The model under review builds one solid part; all positions refer to its coordinate system, in mm. Face numbers are marked on the shaded views. A direction names the side the tool comes from. Round coordinates to 2 decimals unless told otherwise and drop trailing zeros. Write each loop counter-clockwise with the first axis right and the second up, starting at its lowest first coordinate (ties: lowest second). Pieces come first, ordered by that corner, then holes. Notation, with made-up numbers: (46.25, -16) - (91.25, -16) arc R19 ccw to (91.25, 8) - close; hole circle Ø8 at (6, -24.75). An arc over 180 degrees is marked (long way). Return JSON: item names as keys, results as strings.
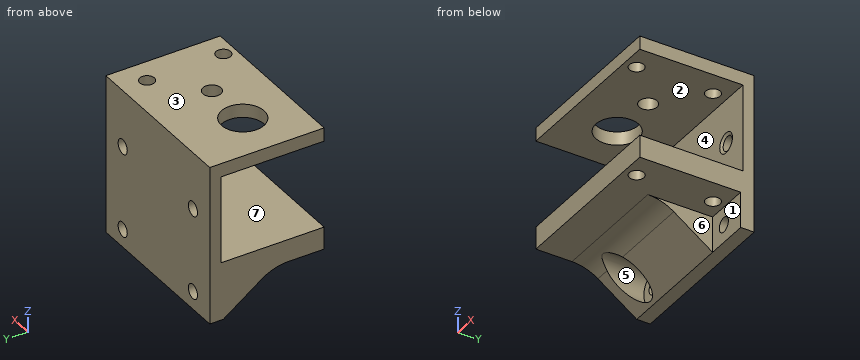
from build123d import *

# Parameters (mm, degrees)
BOSS_EXTRUDE1_OUTLINE_W   = 37
BOSS_EXTRUDE1_OUTLINE_H   = 22.5
BOSS_EXTRUDE1_OUTLINE_R   = 1.625
BOSS_EXTRUDE1_OUTLINE_R_2 = 4.75
BOSS_EXTRUDE1_OUTLINE_R_3 = 2
BOSS_EXTRUDE1_DEPTH       = 3
SKETCH2_W                 = 37
SKETCH2_H                 = 22.5
SKETCH2_R                 = 1.625
BOSS_EXTRUDE2_DEPTH       = 5
SKETCH3_W                 = 37
SKETCH3_H                 = 35.5
BOSS_EXTRUDE3_DEPTH       = 3
BOSS_EXTRUDE4_DEPTH       = 37
CUT_EXTRUDE1_DEPTH        = 10
CUT_EXTRUDE2_REACH        = 57.457
SKETCH7_R                 = 1.625
CHAMFER1_SIZE             = 1.5
CHAMFER1_SIZE2            = 0.866025404
FILLET1_R                 = 10
SKETCH8_R                 = 3.5
CUT_EXTRUDE3_DEPTH        = 22.5
SKETCH9_W                 = 37
SKETCH9_H                 = 19.5
CUT_EXTRUDE4_DEPTH        = 0.5


# Read off the part's stored shape, not the designer's step: Boss-Extrude1
with BuildPart() as part:
    # Boss-Extrude1 outline → Boss-Extrude1 (new body)
    with BuildSketch(Plane.XY):
        with Locations((18.5, 11.25)):
            Rectangle(BOSS_EXTRUDE1_OUTLINE_W, BOSS_EXTRUDE1_OUTLINE_H)
        with Locations((31.5, 2.75)):
            Circle(BOSS_EXTRUDE1_OUTLINE_R, mode=Mode.SUBTRACT)
        with Locations((11, 11.25)):
            Circle(BOSS_EXTRUDE1_OUTLINE_R_2, mode=Mode.SUBTRACT)
        with Locations((22, 11.25)):
            Circle(BOSS_EXTRUDE1_OUTLINE_R_3, mode=Mode.SUBTRACT)
        with Locations((31.5, 19.75)):
            Circle(BOSS_EXTRUDE1_OUTLINE_R, mode=Mode.SUBTRACT)
    extrude(amount=BOSS_EXTRUDE1_DEPTH)



with BuildPart() as body_2:
    # Sketch2 → Boss-Extrude2 (new body)
    with BuildSketch(Plane(origin=(0, 0, -19.5), x_dir=(-1, 0, 0), z_dir=(0, 0, -1))):
        with Locations((-18.5, 11.25)):
            Rectangle(SKETCH2_W, SKETCH2_H)
        with Locations((-31.5, 2.75)):
            Circle(SKETCH2_R, mode=Mode.SUBTRACT)
        with Locations(Location((-31.5, 19.75, 0), (0, 0, 180))):
            Circle(SKETCH2_R, mode=Mode.SUBTRACT)
    extrude(amount=BOSS_EXTRUDE2_DEPTH)


with BuildPart() as part_1:
    add(part.part)

    add(body_2.part)  # Boss-Extrude3 merges body 2
    # Sketch3 → Boss-Extrude3 (add)
    with BuildSketch(Plane.XZ.offset(-22.5)):
        with Locations((18.5, -14.75)):
            Rectangle(SKETCH3_W, SKETCH3_H)
    extrude(amount=-BOSS_EXTRUDE3_DEPTH)

    # Sketch6 → Boss-Extrude4 (add)
    with BuildSketch(Plane(origin=(37, 0, 0), x_dir=(0, 0, -1), z_dir=(1, 0, 0))):
        Polygon((32.5, 22.5), (24.5, 11.25), (24.5, 22.5), align=None)
    extrude(amount=-BOSS_EXTRUDE4_DEPTH)

    # Sketch6<2> → Cut-Extrude1 (cut)
    with BuildSketch(Plane(origin=(37, 0, 0), x_dir=(0, 0, -1), z_dir=(1, 0, 0))):
        Polygon((32.5, 22.5), (24.5, 11.25), (24.5, 22.5), align=None)
    extrude(amount=-CUT_EXTRUDE1_DEPTH, mode=Mode.SUBTRACT)

    # Sketch7 → Cut-Extrude2 (cut, up to next)
    with BuildSketch(Plane(origin=(0, 25.5, 0), x_dir=(-1, 0, 0), z_dir=(0, 1, 0)), mode=Mode.PRIVATE) as cut_extrude2_sk1:
        with Locations(Location((-6, -9.75, 0), (0, 0, 90))):
            Circle(SKETCH7_R)
    cut_extrude2_tool1 = extrude(cut_extrude2_sk1.sketch, amount=-CUT_EXTRUDE2_REACH, mode=Mode.PRIVATE) & part_1.part
    # Sketch7 → Cut-Extrude2 (cut, up to next)
    with BuildSketch(Plane(origin=(0, 25.5, 0), x_dir=(-1, 0, 0), z_dir=(0, 1, 0)), mode=Mode.PRIVATE) as cut_extrude2_sk2:
        with Locations(Location((-31, -9.75, 0), (0, 0, 90))):
            Circle(SKETCH7_R)
    cut_extrude2_tool2 = extrude(cut_extrude2_sk2.sketch, amount=-CUT_EXTRUDE2_REACH, mode=Mode.PRIVATE) & part_1.part
    # Sketch7 → Cut-Extrude2 (cut, up to next)
    with BuildSketch(Plane(origin=(0, 25.5, 0), x_dir=(-1, 0, 0), z_dir=(0, 1, 0)), mode=Mode.PRIVATE) as cut_extrude2_sk3:
        with Locations(Location((-6, -28.5, 0), (0, 0, 90))):
            Circle(SKETCH7_R)
    cut_extrude2_tool3 = extrude(cut_extrude2_sk3.sketch, amount=-CUT_EXTRUDE2_REACH, mode=Mode.PRIVATE) & part_1.part
    # Sketch7 → Cut-Extrude2 (cut, up to next)
    with BuildSketch(Plane(origin=(0, 25.5, 0), x_dir=(-1, 0, 0), z_dir=(0, 1, 0)), mode=Mode.PRIVATE) as cut_extrude2_sk4:
        with Locations(Location((-31, -28.5, 0), (0, 0, 90))):
            Circle(SKETCH7_R)
    cut_extrude2_tool4 = extrude(cut_extrude2_sk4.sketch, amount=-CUT_EXTRUDE2_REACH, mode=Mode.PRIVATE) & part_1.part
    add(cut_extrude2_tool1.solids().sort_by_distance((6, 25.5, -9.75))[0], mode=Mode.SUBTRACT)
    add(cut_extrude2_tool2.solids().sort_by_distance((31, 25.5, -9.75))[0], mode=Mode.SUBTRACT)
    add(cut_extrude2_tool3.solids().sort_by_distance((6, 25.5, -28.5))[0], mode=Mode.SUBTRACT)
    add(cut_extrude2_tool4.solids().sort_by_distance((31, 25.5, -28.5))[0], mode=Mode.SUBTRACT)

    # Chamfer1
    chamfer1_edges = [part_1.edges().sort_by_distance(p)[0] for p in [
        (31, 22.5, -11.375),
        (6, 22.5, -11.375),
    ]]
    chamfer1_side = [part_1.faces().sort_by_distance(p)[0] for p in [
        (18.5, 22.5, -9.75),
    ]]
    chamfer(chamfer1_edges, length=CHAMFER1_SIZE, length2=CHAMFER1_SIZE2, reference=chamfer1_side[0])

    # Fillet1
    fillet1_edges = [part_1.edges().sort_by_distance(p)[0] for p in [
        (13.5, 11.25, -24.5),
    ]]
    fillet(fillet1_edges, radius=FILLET1_R)

    # Sketch8 → Cut-Extrude3 (cut)
    with BuildSketch(Plane(origin=(0, 0, 0), x_dir=(1, 0, 0), z_dir=(0, 1, 0))):
        with Locations(Location((6, 28.5, 0), (0, 0, 322.109230385))):
            Circle(SKETCH8_R)
    extrude(amount=CUT_EXTRUDE3_DEPTH, mode=Mode.SUBTRACT)

    # Sketch9 → Cut-Extrude4 (cut)
    with BuildSketch(Plane(origin=(0, 22.5, 0), x_dir=(-1, 0, 0), z_dir=(0, -1, 0))):
        with Locations((-18.5, 9.75)):
            Rectangle(SKETCH9_W, SKETCH9_H)
    extrude(amount=-CUT_EXTRUDE4_DEPTH, mode=Mode.SUBTRACT)


solid = part_1.part
(1) Clearance check with flat-ended pins moving along their axes: pin 1 Ø4 at (x, y) = (31.5, 19.75) entering from -Z; pin 2 Ø12.5 at (x, y) = (11, 11.25) entering from -Z; pin 3 Ø2.5 at (x, y) = (31.5, 2.75) entering from +Z; pin 4 Ø6.5 at (y, z) = (18.5, -28.5) entering from +X. State where each tip first meets the part, or that it passes through.
Filled in:
{"pin 1": "stops at z = -24.5", "pin 2": "stops at z = -28.94", "pin 3": "passes through", "pin 4": "stops at x = 27"}
(2) Add section B-B (z = -9.75). Write out the cut boundary in (x, y) (3 decimals), plus the area to 3 significant figures.
Filled in:
{"outline": "(0, 23) - (3.741, 23) - (4.375, 23.366) - (4.375, 25.5) - (0, 25.5) - close; (7.625, 23.366) - (8.259, 23) - (28.741, 23) - (29.375, 23.366) - (29.375, 25.5) - (7.625, 25.5) - close; (32.625, 23.366) - (33.259, 23) - (37, 23) - (37, 25.5) - (32.625, 25.5) - close", "area": "75.8 mm2"}
(3) Add section A-A (x = 22). Write out the cut boundary in (y, z).
Filled in:
{"outline": "(0, -24.5) - (8.06, -24.5) arc R10 cw to (13.85, -26.35) - (22.5, -32.5) - (25.5, -32.5) - (25.5, 3) - (13.25, 3) - (13.25, 0) - (23, 0) - (23, -19.5) - (0, -19.5) - close; (0, 0) - (9.25, 0) - (9.25, 3) - (0, 3) - close"}
(4) Add section D-D (x = 13). Write out the cut boundary in (y, z), plus the area to 3 significant figures.
Filled in:
{"outline": "(0, -24.5) - (8.06, -24.5) arc R10 cw to (13.85, -26.35) - (22.5, -32.5) - (25.5, -32.5) - (25.5, 3) - (15.56, 3) - (15.56, 0) - (23, 0) - (23, -19.5) - (0, -19.5) - close; (0, 0) - (6.94, 0) - (6.94, 3) - (0, 3) - close", "area": "297 mm2"}
(5) Add section C-C (y = 11.75). Write out the cut boundary in (x, z).
Filled in:
{"outline": "(0, -25.21) - (4.81, -25.21) arc R3.5 cw to (7.19, -25.21) - (27, -25.21) - (27, -24.5) - (37, -24.5) - (37, -19.5) - (0, -19.5) - close; (0, 0) - (6.28, 0) - (6.28, 3) - (0, 3) - close; (15.72, 0) - (20.06, 0) - (20.06, 3) - (15.72, 3) - close; (23.94, 0) - (37, 0) - (37, 3) - (23.94, 3) - close"}
(6) For the marked faces 5, 6 and 7, list the 3-axis set-ups (+Z, -Z, +X, -X, +Y, -Y) from which the entire face can be reached by the end or side of a thin tool; tool diameter is ignored.
Filled in:
{"face 5": "-Y", "face 6": "-Z, +X, -Y", "face 7": "+X, -X, -Y"}
(7) Wall thickness on line 1 (Z direction, x = 34, y = 1); line 2 (Y direction, x = 31.5, z = -22.9) (3 decimals); line 3 (Y direction, x = 31, z = -21): over which ranges is each line inside the solid? List them lowest first.
Filled in:
{"line 1": "z = -24.5 to -19.5, 0 to 3", "line 2": "y = 0 to 1.125, 4.375 to 18.125, 21.375 to 25.5", "line 3": "y = 0 to 1.2, 4.3 to 18.2, 21.3 to 25.5"}
(8) Mouldability with a two-part tool opening along Z and no side actions: class the marked faces 1, 2, 3 and 4 as released by +Z, released by -Z, zero draft, split by the parting line, or undercut.
Filled in:
{"face 1": "zero draft", "face 2": "undercut", "face 3": "released by +Z", "face 4": "undercut"}
